Model file for the job. Use its own axes, mm. A direction names the side the tool comes from. Give positions to 0.01 mm unless a question says otherwise; leave off trailing zeros. Loops run counter-clockwise (first coordinate to the right, second up) from the corner with the lowest first, then second, coordinate; pieces in that order, holes last. Notation, with made-up numbers: M 57.25,-34 L 85.25,-34 A15 cw 85.25,-30 Z; hole C 17,39 d5. An arc over 180 degrees is marked long. Answer in a Markdown table with one row per item.
```python
from build123d import *

# Parameters (mm, degrees)
SWEEP1_PROFILE_R     = 12.7
SWEEP2_PROFILE_R     = 12.7
SWEEP3_PROFILE_R     = 12.7
CUT_SWEEP1_START     = -81.549620248
CUT_SWEEP1_OUTLINE_W = 67
CUT_SWEEP1_OUTLINE_H = 33
CUT_SWEEP1_DEPTH     = 44.599672867


# Read off the part's stored shape, not the designer's step: Cut-Sweep1
with BuildPart() as part:
    # Sweep1: sweep along a path in Sketch1
    with BuildLine(Plane.XY) as sweep1_path:
        Line((275.126088043, -73.014540772), (239.071642227, -37.227435037))
        Line((239.071642227, -37.227435037), (193.952445621, 7.557207275))
        ThreePointArc((193.952445621, 7.557207275), (174.105035635, 19.737252225), (150.908197029, 21.781722044))
        Line((150.908197029, 21.781722044), (7.257142857, 1.047478346))
        ThreePointArc((7.257142857, 1.047478346), (0, 0.526438931), (-7.257142857, 1.047478346))
        Line((-7.257142857, 1.047478346), (-150.908197029, 21.781722044))
        ThreePointArc((-150.908197029, 21.781722044), (-174.105035635, 19.737252225), (-193.952445621, 7.557207275))
        Line((-193.952445621, 7.557207275), (-239.071642227, -37.227435037))
        Line((-239.071642227, -37.227435037), (-275.126088043, -73.014540772))
    # Sweep1 profile (on start of the path) → Sweep1 (sweep)
    with BuildSketch(Plane(origin=(275.126088043, -73.014540772, 0), x_dir=(-0.7044705853386212, -0.7097331853539472, 0), z_dir=(-0.7097331853539472, 0.7044705853386212, 0))):
        Circle(SWEEP1_PROFILE_R)
    sweep(path=sweep1_path.line)

    # Sweep2: sweep along a path in Sketch1<3>
    with BuildLine(Plane.XY) as sweep2_path:
        Line((109.5375, 15.810376278), (109.5375, 241.235376278))
    # Sweep2 profile (on start of the path) → Sweep2 (sweep)
    with BuildSketch(Plane(origin=(109.5375, 15.810376278, 0), x_dir=(0, 0, 1), z_dir=(0, 1, 0))):
        Circle(SWEEP2_PROFILE_R)
    sweep2 = sweep(path=sweep2_path.line)

    # Sweep3: sweep along a path in Sketch1<4>
    with BuildLine(Plane.XY) as sweep3_path:
        Line((128.5875, 241.235376278), (90.4875, 241.235376278))
    # Sweep3 profile (on start of the path) → Sweep3 (sweep)
    with BuildSketch(Plane(origin=(128.5875, 241.235376278, 0), x_dir=(0, -1, 0), z_dir=(-1, 0, 0))):
        Circle(SWEEP3_PROFILE_R)
    sweep3 = sweep(path=sweep3_path.line)

    # Cut-Sweep1 outline → Cut-Sweep1 (cut)
    with BuildSketch(Plane(origin=(0, 0, 0), x_dir=(1, 0, 0), z_dir=(0, 0.992546151641322, 0.121869343405149)).offset(CUT_SWEEP1_START)):
        with Locations((252.5, -6.5)):
            Rectangle(CUT_SWEEP1_OUTLINE_W, CUT_SWEEP1_OUTLINE_H)
    cut_sweep1 = extrude(amount=CUT_SWEEP1_DEPTH, mode=Mode.SUBTRACT)

    # Mirror2: Sweep2, Sweep3, Cut-Sweep1 across plane
    add(sweep2.mirror(Plane(origin=(0, 0, 0), x_dir=(0, 0, 1), z_dir=(1, 0, 0))))
    add(sweep3.mirror(Plane(origin=(0, 0, 0), x_dir=(0, 0, 1), z_dir=(1, 0, 0))))
    add(cut_sweep1.mirror(Plane(origin=(0, 0, 0), x_dir=(0, 0, 1), z_dir=(1, 0, 0))), mode=Mode.SUBTRACT)


solid = part.part
```
Q1. Probe probe 1 along X at (y, z) = (236, -3.5); probe 2 along X at (y, z) = (46, 0.5); probe 3 along Z at (x, y) = (11.5, 1.5). List the from-to ranges inside material, lowest first.
Reported:
| item | result |
|---|---|
| probe 1 | -128.59 to -90.49, 90.49 to 128.59 |
| probe 2 | -122.23 to -96.85, 96.85 to 122.23 |
| probe 3 | -12.7 to 12.7 |
Q2. Mould opens along X. For faces 5 (the face through (128.588, 241, 0)), 6 (the face through (-238.818, -37.206, -0.178)), 7 (the face through (-81.82, -0.43, 3.81)), 8 (the face through (-98.27, 130.1, 5.86)) say: released by +X, released by -X, zero draft, split by the parting line, or undercut.
Reported:
| item | result |
|---|---|
| face 5 | released by +X |
| face 6 | zero draft |
| face 7 | undercut |
| face 8 | undercut |
Q3. Drop flat-ended pins along their axis: pin 1 (1 mm diameter, centred on x = -8.5, z = 6.5, fed in from -Y); pin 2 (2 mm diameter, centred on x = 169, z = -3, fed in from +Y); pin 3 (4 mm diameter, centred on y = 120, z = -7.5, fed in from -X). Give the stop position or say it passes through.
Reported:
| item | result |
|---|---|
| pin 1 | y = -10.09 |
| pin 2 | y = 33.98 |
| pin 3 | x = -120.98 |
Q4. 3-axis set-ups, long thin cutter, end or side, ignore diameter. For faces 1 (the face through (-90.488, 241, 0)), 2 (the face through (109.271, 253.923, 0.558)), 3 (the face through (-128.588, 241, 0)), 4 (the face through (238.818, -37.206, -0.178)): which of +Z, -Z, +X, -X, +Y, -Y reach the whole face in a straight line?
Reported:
| item | result |
|---|---|
| face 1 | +Z, -Z, +Y |
| face 2 | none |
| face 3 | +Z, -Z, -X, +Y |
| face 4 | -Z, +X, -X, -Y |
Q5. Saw through at B-B (y = 174). Give the cut face in (x, z), and give its area (3 significant figures).
Reported:
| item | result |
|---|---|
| outline | C -109.54,0 d25.4; C 109.54,0 d25.4 |
| area | 1,010 mm² |
